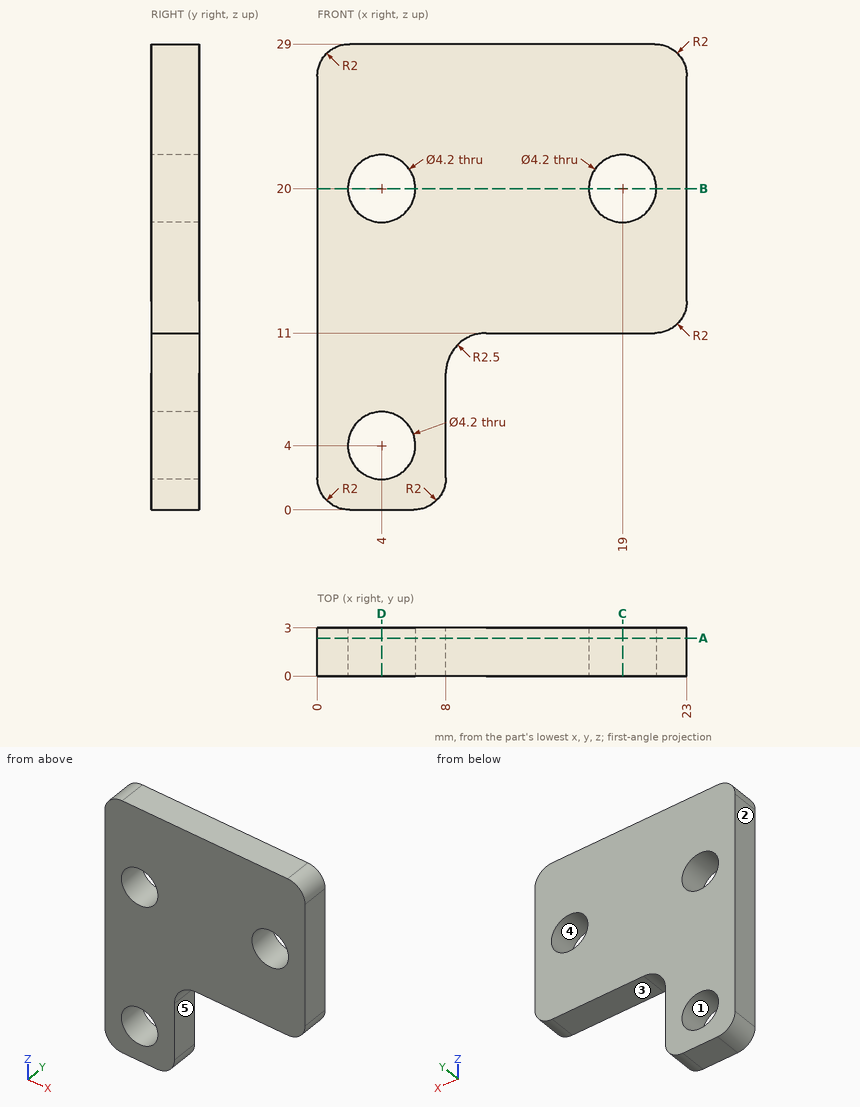
Could you check a few things on this drawing? It's one solid part, dimensions in mm from its lowest x, y, z. A direction names the side the tool comes from. Round coordinates to 2 decimals unless told otherwise and drop trailing zeros. Loops run counter-clockwise (first coordinate to the right, second up) from the corner with the lowest first, then second, coordinate; pieces in that order, holes last. Notation, with made-up numbers: (67.25, 3.25) -> (88.25, 3.25) arc R23 cw to (88.25, 12.25) -> close; hole circle Ø2 at (-19.5, -1.75). An arc over 180 degrees is marked (long way). Write each question's results on one line, items separated by ' | '.
(1) For the marked faces 4 and 5, which set-ups out of +Z, -Z, +X, -X, +Y, -Y let a thin tool reach every point of the face, with its end or its side?
Worked answers:
face 4: +Y, -Y | face 5: -Z, +X, +Y, -Y
(2) If we section it at B-B, the plane z = 20: List the corners of the cut face in (x, y) for me.
Worked answers:
outline: (0, 0) -> (1.9, 0) -> (1.9, 3) -> (0, 3) -> close; (6.1, 0) -> (16.9, 0) -> (16.9, 3) -> (6.1, 3) -> close; (21.1, 0) -> (23, 0) -> (23, 3) -> (21.1, 3) -> close
(3) If we section it at D-D, the plane x = 4: List the corners of the cut face in (y, z) for me, then the cut area to 3 significant figures.
Worked answers:
outline: (0, 0) -> (3, 0) -> (3, 1.9) -> (0, 1.9) -> close; (0, 6.1) -> (3, 6.1) -> (3, 17.9) -> (0, 17.9) -> close; (0, 22.1) -> (3, 22.1) -> (3, 29) -> (0, 29) -> close | area: 61.8 mm2
(4) We'd pull the mould along Z, two halves only. Please class the marked faces 1, 2 and 3: released by +Z, released by -Z, zero draft, split by the parting line, or undercut.
Worked answers:
face 1: undercut | face 2: zero draft | face 3: released by -Z
(5) If we section it at C-C, the plane x = 19: List the corners of the cut face in (y, z) for me, then the cut area to 3 significant figures.
Worked answers:
outline: (0, 11) -> (3, 11) -> (3, 17.9) -> (0, 17.9) -> close; (0, 22.1) -> (3, 22.1) -> (3, 29) -> (0, 29) -> close | area: 41.4 mm2
(6) If we section it at A-A, the plane y = 2.35: List the corners of the cut face in (x, z) for me.
Worked answers:
outline: (0, 2) arc R2 ccw to (2, 0) -> (6, 0) arc R2 ccw to (8, 2) -> (8, 8.5) arc R2.5 cw to (10.5, 11) -> (21, 11) arc R2 ccw to (23, 13) -> (23, 27) arc R2 ccw to (21, 29) -> (2, 29) arc R2 ccw to (0, 27) -> close; hole circle Ø4.2 at (4, 4); hole circle Ø4.2 at (4, 20); hole circle Ø4.2 at (19, 20)
(7) For P1, Ø3.5, axis at x = 4, z = 4, coming from the -Y side; P2, Ø10, axis at x = 5.5, z = 10.5, coming from the -Y side; P3, Ø0.9, axis at y = 1.5, z = 6, coming from the +X side; P4, Ø1.5, axis at x = 18, y = 1.5, coming from the -Z side, each with a flat end and sliding along its axis, tell me the tip position at first contact or that it passes through.
Worked answers:
P1: through | P2: y = 0 | P3: x = 8 | P4: z = 11
(8) If I drill on L1, parallel to X at y = 2, z = 20; L2, parallel to Z at x = 4, y = 1.25; L3, parallel to Z at x = 19, y = 1.35, over which ranges is the centre line in solid material (lowest first)?
Worked answers:
L1: 0 to 1.9, 6.1 to 16.9, 21.1 to 23 | L2: 0 to 1.9, 6.1 to 17.9, 22.1 to 29 | L3: 11 to 17.9, 22.1 to 29
